Read the model definition and answer for the solid it produces. Units are mm, in the model's axes. A direction names the side the tool comes from. Round coordinates to 2 decimals unless told otherwise and drop trailing zeros. Order: outer loops, then holes, each group sorted by start corner. A loop starts at its lowest first (then second) coordinate and runs counter-clockwise, first axis right, second up. Notation, with made-up numbers: (-21.75, 49.25) - (-17.75, 49.25) arc R35 cw to (-17.75, 83.25) - close; hole circle Ø1 at (84, 5). An arc over 180 degrees is marked (long way). Answer as a JSON object with one key per item and string values. Group by question number.
Q1. A tool of negligible diameter and unlimited length cuts with its end or side. For faces 1 (the flat face through (-4.54, -38.98, 0.99)), 2 (the flat face through (0, 46, 1)), 3 (the flat face through (-3, 41.5, 1)), from which of +Z, -Z, +X, -X, +Y, -Y can it reach the whole face along a straight path? Write none if from no direction.
Q2. Consider line 1 (Y direction, x = -3, z = 1.3); line 2 (Y direction, x = -3, z = 0.95); line 3 (X direction, y = -17, z = 1.95). Determine where each line is inside the solid, lowest interval first.
Q3. A cutting plane is placed at D-D on x = -8. Determine the outline of the cut face in (y, z), and give its area (3 significant figures).
Q4. A cutting plane is placed at B-B on y = -40.5. Determine the outline of the cut face in (x, z), and give its area (3 significant figures).
Q5. The mould has two halves that part along Y. Classify faces 4 (the flat face through (-8.427, -35.482, 0.986)), 5 (the flat face through (-10.1, 49.1, 0.9)), 6 (the flat face through (-12, 1, 2)): pulls with the +Y half, pulls with the -Y half, needs draft (parallel to the pull), parting line crosses it, or undercut.
Q6. A cutting plane is placed at C-C on x = -15. Determine the outline of the cut face in (y, z), and give its area (3 significant figures).
Q7. Given pin 1 Ø12 at (x, y) = (-2.5, 33.5) entering from -Z; pin 2 Ø0.6 at (x, z) = (-2, 1) entering from -Y, each flat-ended and moving along its own axis, determine where each tip first touches the part or whether it passes through.
```python
from build123d import *

# Parameters (mm, degrees)
SKETCH_W     = 40
SKETCH_H     = 100
SKETCH_R     = 2.5
PAD_DEPTH    = 2
CHAMFER_SIZE = 1.8
BOX_W        = 22
BOX_H        = 119
BOX_DEPTH    = 7
BOX001_W     = 5
BOX001_H     = 9
BOX001_DEPTH = 2


with BuildPart() as part:
    # Sketch → Pad (new body)
    with BuildSketch(Plane.XY):
        Rectangle(SKETCH_W, SKETCH_H)
        with Locations((-8, -40.5)):
            Circle(SKETCH_R, mode=Mode.SUBTRACT)
        with Locations((8, 40.5)):
            Circle(SKETCH_R, mode=Mode.SUBTRACT)
        Polygon((6.5, -41.5), (6.5, 36.5), (0, 36.5), (0, 41.5), (-6.5, 41.5), (-6.5, -36.5), (0, -36.5), (0, -41.5), align=None, mode=Mode.SUBTRACT)
    extrude(amount=PAD_DEPTH)

    # Chamfer
    chamfer_edges = [part.edges().sort_by_distance(p)[0] for p in [
        (-20, 0, 0),
        (0, -50, 0),
        (20, 0, 0),
        (0, 50, 0),
    ]]
    chamfer(chamfer_edges, length=CHAMFER_SIZE)

    # Box → Box (cut)
    with BuildSketch(Plane(origin=(0, 58, 4), x_dir=(1, 0, 0), z_dir=(0, 0, -1))):
        with Locations((11, 59.5)):
            Rectangle(BOX_W, BOX_H)
    extrude(amount=BOX_DEPTH, mode=Mode.SUBTRACT)

    # Box001 → Box001 (cut)
    with BuildSketch(Plane(origin=(-10.3, -39.5, 0), x_dir=(0.906308, -0.422618, 0), z_dir=(0, 0, 1))):
        with Locations((2.5, 4.5)):
            Rectangle(BOX001_W, BOX001_H)
    extrude(amount=BOX001_DEPTH, mode=Mode.SUBTRACT)


solid = part.part
```
Result set:
{
 "1": {"face 1": "+Z, -Z", "face 2": "+Z, -Z, +X, +Y, -Y", "face 3": "+Z, -Z, +X"},
 "2": {"line 1": "y = -49.5 to -36.5, 41.5 to 49.5", "line 2": "y = -49.15 to -36.5, 41.5 to 49.15", "line 3": "x = -20 to -6.5"},
 "3": {"outline": "(-50, 1.8) - (-48.2, 0) - (-43, 0) - (-43, 2) - (-50, 2) - close; (-34.57, 0) - (48.2, 0) - (50, 1.8) - (50, 2) - (-34.57, 2) - close", "area": "180 mm²"},
 "4": {"outline": "(-20, 1.8) - (-18.2, 0) - (-10.5, 0) - (-10.5, 2) - (-20, 2) - close; (-5.25, 0) - (0, 0) - (0, 2) - (-5.25, 2) - close", "area": "27.9 mm²"},
 "5": {"face 4": "undercut", "face 5": "pulls with the +Y half", "face 6": "needs draft"},
 "6": {"outline": "(-50, 1.8) - (-48.2, 0) - (48.2, 0) - (50, 1.8) - (50, 2) - (-50, 2) - close", "area": "197 mm²"},
 "7": {"pin 1": "stops at z = 0", "pin 2": "stops at y = -49.5"}
}
